Here's the drawing with two shaded views (mm, measured from the low corner). I have some questions. A direction names the side the tool comes from. Give positions to 0.01 mm unless a question says otherwise; leave off trailing zeros. Write each loop counter-clockwise with the first axis right and the second up, starting at its lowest first coordinate (ties: lowest second). Pieces come first, ordered by that corner, then holes. Notation, with made-up numbers: (49.5, 28) -> (93.5, 28) arc R31 cw to (93.5, 64) -> close; hole circle Ø9 at (45.5, 57.5). An arc over 180 degrees is marked (long way). One line per item, written item: value.
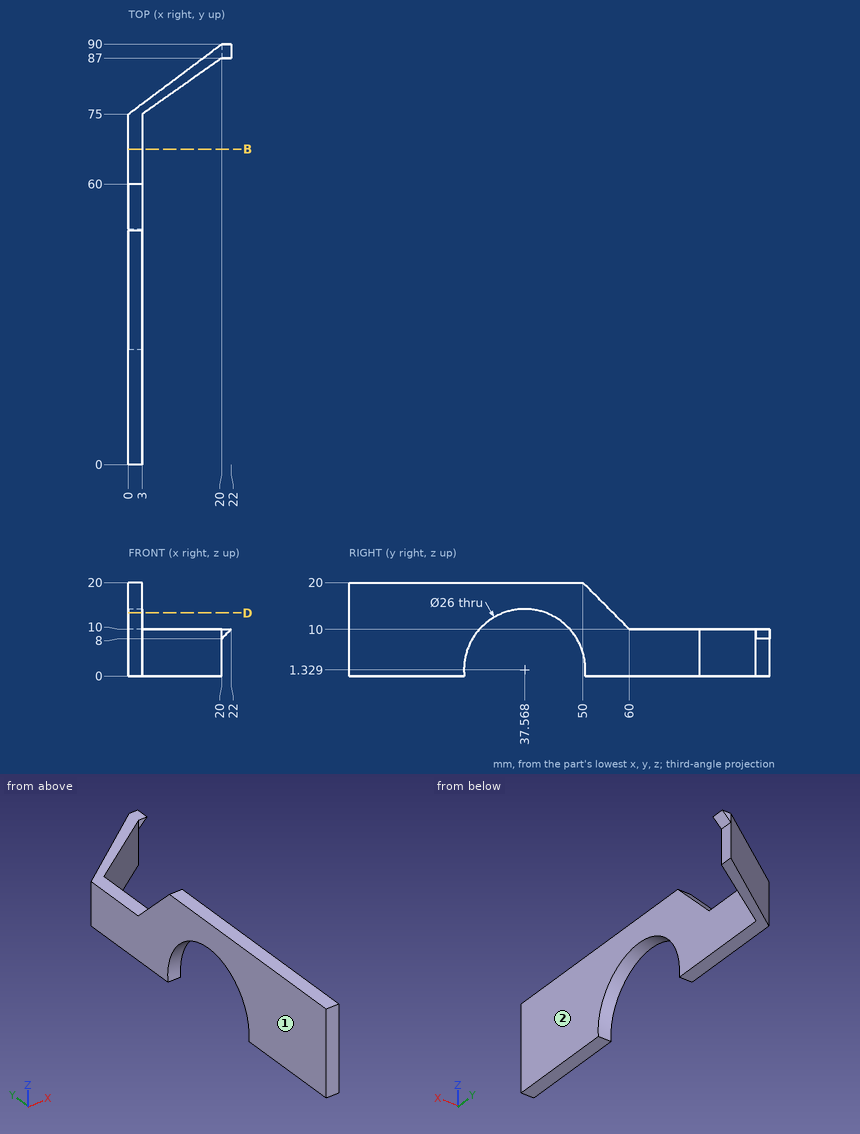
1) If we section it at D-D (z = 13.5): Write out the boundary of the cut face in (x, y), and give its area (3 significant figures).
Answer list:
outline: (0, 0) -> (3, 0) -> (3, 33) -> (0, 33) -> close; (0, 42.14) -> (3, 42.14) -> (3, 56.5) -> (0, 56.5) -> close
area: 142 mm^2
2) I need wall thicknesses on L1, parallel to X at y = 68, z = 1.75; L2, parallel to Y at x = 1, z = 17.75; L3, parallel to Y at x = 4.25, z = 9. Which ranges of each line are inside material? Lowest first, please.
Answer list:
L1: x = 0 to 3
L2: y = 0 to 52.25
L3: y = 75.88 to 78.19
3) For the marked faces 1 and 2, which set-ups out of +Z, -Z, +X, -X, +Y, -Y let a thin tool reach every point of the face, with its end or its side?
Answer list:
face 1: +Z, -Z, -X, +Y, -Y
face 2: +Z, -Z, +X, -Y
4) If we section it at B-B (y = 67.5): Write out the boundary of the cut face in (x, z), and give its area (3 significant figures).
Answer list:
outline: (0, 0) -> (3, 0) -> (3, 10) -> (0, 10) -> close
area: 30.0 mm^2
5) Will these pins go through, and if not, where does the flat tip stop? pin 1 (2.5 mm diameter, centred on y = 89, z = 2.5, fed in from +X); pin 2 (10 mm diameter, centred on y = 51.5, z = 12, fed in from +X); pin 3 (3 mm diameter, centred on y = 49.5, z = 14.5, fed in from -X); pin 4 (6 mm diameter, centred on x = 12, z = 12.5, fed in from +Y) (1 decimal).
Answer list:
pin 1: stops at x = 20
pin 2: stops at x = 3
pin 3: stops at x = 0
pin 4: stops at y = 85.2
